Part model, mm, in its own coordinate system. Face numbers are marked on the shaded views. A direction names the side the tool comes from. Round coordinates to 2 decimals unless told otherwise and drop trailing zeros. Loops run counter-clockwise (first coordinate to the right, second up) from the corner with the lowest first, then second, coordinate; pieces in that order, holes last.
(1) Cut at A-A on x = 6. List the corners of the cut face in (y, z).
(2) Probe probe 1 along Z at (x, y) = (-13.5, -1.75); probe 2 along Y at (x, z) = (16, 2.25); probe 3 along X at (y, z) = (-3.5, 2.75). List the from-to ranges inside material, lowest first.
(3) Cut at B-B on y = 6.25. List the corners of the cut face in (x, z).
(4) Tool access for the marked faces 1, 2 and 3: list every direction of +Z, -Z, +X, -X, +Y, -Y with a clear straight run to the whole face (end or side of a thin tool).
(5) Cut at D-D on x = -4. List the corners of the cut face in (y, z), then the cut area to 3 significant figures.
(6) Flat gauge pins, fed straight in: pin 1 (5.5 mm diameter, centred on y = 1.5, z = 9, fed in from +X); pin 2 (6 mm diameter, centred on x = 15, z = 8.5, fed in from +Y); pin 3 (2.5 mm diameter, centred on x = -7, z = 8.5, fed in from -Y); pin 4 (3 mm diameter, centred on x = -7.5, z = 8.5, fed in from +Y). Where does each tip first touch, or does it go through?
(7) Cut at C-C on z = 10.75. List the corners of the cut face in (x, y), then the cut area to 3 significant figures.
from build123d import *

# Parameters (mm, degrees)
F0_W     = 54
F0_H     = 22.4
F0_W_2   = 5
F0_H_2   = 5
F1_DEPTH = 2
F2_DEPTH = 13
F3_DEPTH = 3.5
F4_R     = 2


# Not quite as in the source:
# - a feature names something its author has since deleted; it is built from what else it names


with BuildPart() as f1:
    # F0 (on Top) → F1 (new body)
    with BuildSketch(Plane.XY):
        with Locations((1.3893617413, 0.829365923)):
            Rectangle(F0_W, F0_H)
        Polygon((-23.1106382587, 3.1091097071), (-23.1106382587, 9.529365923), (25.8893617413, 9.529365923), (25.8893617413, 3.079365923), (25.8893617413, 0.829365923), (25.8893617413, -1.420634077), (25.8893617413, -7.870634077), (-23.1106382587, -7.870634077), (-23.1106382587, -1.3557597995), (-23.1106382587, 0.859365923), align=None, mode=Mode.SUBTRACT)
        with BuildLine():
            Line((25.8893617413, 9.529365923), (-23.1106382587, 9.529365923))
            Line((-23.1106382587, 9.529365923), (-23.1106382587, 3.1091097071))
            Line((-23.1106382587, 3.1091097071), (-20.8945927259, 3.1091097071))
            ThreePointArc((-20.8945927259, 3.1091097071), (-19.2816983534, 2.4623159458), (-18.6106382587, 0.859365923))
            ThreePointArc((-18.6106382587, 0.859365923), (-19.4158848712, -0.8655073041), (-21.2552495026, -1.3557597995))
            Line((-21.2552495026, -1.3557597995), (-23.1106382587, -1.3557597995))
            Line((-23.1106382587, -1.3557597995), (-23.1106382587, -7.870634077))
            Line((-23.1106382587, -7.870634077), (25.8893617413, -7.870634077))
            Line((25.8893617413, -7.870634077), (25.8893617413, -1.420634077))
            Line((25.8893617413, -1.420634077), (23.6393617413, -1.420634077))
            ThreePointArc((23.6393617413, -1.420634077), (21.3893617413, 0.829365923), (23.6393617413, 3.079365923))
            Line((23.6393617413, 3.079365923), (25.8893617413, 3.079365923))
            Line((25.8893617413, 3.079365923), (25.8893617413, 9.529365923))
        make_face()
        with Locations((-5.8658428788, 0.829365923)):
            Rectangle(F0_W_2, F0_H_2, mode=Mode.SUBTRACT)
        with BuildLine():
            Line((-20.8945927259, 3.1091097071), (-23.1106382587, 3.1091097071))
            Line((-23.1106382587, 3.1091097071), (-23.1106382587, 0.859365923))
            ThreePointArc((-23.1106382587, 0.859365923), (-22.4635882815, 2.4383058282), (-20.8945927259, 3.1091097071))
        make_face()
        with BuildLine():
            Line((25.8893617413, 0.829365923), (25.8893617413, 3.079365923))
            Line((25.8893617413, 3.079365923), (23.6393617413, 3.079365923))
            ThreePointArc((23.6393617413, 3.079365923), (25.230351999, 2.4203561806), (25.8893617413, 0.829365923))
        make_face()
        with BuildLine():
            ThreePointArc((-21.2552495026, -1.3557597995), (-22.5855114857, -0.5853874645), (-23.1106382587, 0.859365923))
            Line((-23.1106382587, 0.859365923), (-23.1106382587, -1.3557597995))
            Line((-23.1106382587, -1.3557597995), (-21.2552495026, -1.3557597995))
        make_face()
        with BuildLine():
            ThreePointArc((-20.8945927259, 3.1091097071), (-22.4635882815, 2.4383058282), (-23.1106382587, 0.859365923))
            ThreePointArc((-23.1106382587, 0.859365923), (-22.5855114857, -0.5853874645), (-21.2552495026, -1.3557597995))
            Line((-21.2552495026, -1.3557597995), (-20.8945927259, -1.3557597995))
            Line((-20.8945927259, -1.3557597995), (-20.8945927259, -0.5963975782))
            ThreePointArc((-20.8945927259, -0.5963975782), (-22.8606382587, 0.829365923), (-20.8945927259, 2.2551294242))
            Line((-20.8945927259, 2.2551294242), (-20.8945927259, 3.1091097071))
        make_face()
        with BuildLine():
            ThreePointArc((-18.6106382587, 0.859365923), (-19.2816983534, 2.4623159458), (-20.8945927259, 3.1091097071))
            Line((-20.8945927259, 3.1091097071), (-20.8945927259, 2.2551294242))
            ThreePointArc((-20.8945927259, 2.2551294242), (-20.1463342813, 1.7099713115), (-19.8606382587, 0.829365923))
            ThreePointArc((-19.8606382587, 0.829365923), (-20.1463342813, -0.0512394656), (-20.8945927259, -0.5963975782))
            Line((-20.8945927259, -0.5963975782), (-20.8945927259, -1.3557597995))
            Line((-20.8945927259, -1.3557597995), (-21.2552495026, -1.3557597995))
            ThreePointArc((-21.2552495026, -1.3557597995), (-19.4158848712, -0.8655073041), (-18.6106382587, 0.859365923))
        make_face()
        with BuildLine():
            ThreePointArc((23.6393617413, -1.420634077), (25.230351999, -0.7616243347), (25.8893617413, 0.829365923))
            ThreePointArc((25.8893617413, 0.829365923), (25.230351999, 2.4203561806), (23.6393617413, 3.079365923))
            Line((23.6393617413, 3.079365923), (23.6393617413, 2.2174858052))
            ThreePointArc((23.6393617413, 2.2174858052), (25.043666155, 2.0748896863), (25.7078010014, 0.829365923))
            ThreePointArc((25.7078010014, 0.829365923), (25.043666155, -0.4161578404), (23.6393617413, -0.5587539593))
            Line((23.6393617413, -0.5587539593), (23.6393617413, -1.420634077))
        make_face()
        with BuildLine():
            Line((25.8893617413, -1.420634077), (25.8893617413, 0.829365923))
            ThreePointArc((25.8893617413, 0.829365923), (25.230351999, -0.7616243347), (23.6393617413, -1.420634077))
            Line((23.6393617413, -1.420634077), (25.8893617413, -1.420634077))
        make_face()
        with BuildLine():
            Line((23.6393617413, 2.2174858052), (23.6393617413, 3.079365923))
            ThreePointArc((23.6393617413, 3.079365923), (21.3893617413, 0.829365923), (23.6393617413, -1.420634077))
            Line((23.6393617413, -1.420634077), (23.6393617413, -0.5587539593))
            ThreePointArc((23.6393617413, -0.5587539593), (22.7078010014, 0.829365923), (23.6393617413, 2.2174858052))
        make_face()
        with Locations((-5.8658428788, 0.829365923)):
            Rectangle(F0_W_2, F0_H_2)
    extrude(amount=F1_DEPTH)

    # F0 (on Top) → F2 (join)
    with BuildSketch(Plane.XY):
        with Locations((-5.8658428788, 0.829365923)):
            Rectangle(F0_W_2, F0_H_2)
    extrude(amount=F2_DEPTH)

    # F0 (on Top) → F3 (join)
    with BuildSketch(Plane.XY):
        with BuildLine():
            Line((25.8893617413, 9.529365923), (-23.1106382587, 9.529365923))
            Line((-23.1106382587, 9.529365923), (-23.1106382587, 3.1091097071))
            Line((-23.1106382587, 3.1091097071), (-20.8945927259, 3.1091097071))
            ThreePointArc((-20.8945927259, 3.1091097071), (-19.2816983534, 2.4623159458), (-18.6106382587, 0.859365923))
            ThreePointArc((-18.6106382587, 0.859365923), (-19.4158848712, -0.8655073041), (-21.2552495026, -1.3557597995))
            Line((-21.2552495026, -1.3557597995), (-23.1106382587, -1.3557597995))
            Line((-23.1106382587, -1.3557597995), (-23.1106382587, -7.870634077))
            Line((-23.1106382587, -7.870634077), (25.8893617413, -7.870634077))
            Line((25.8893617413, -7.870634077), (25.8893617413, -1.420634077))
            Line((25.8893617413, -1.420634077), (23.6393617413, -1.420634077))
            ThreePointArc((23.6393617413, -1.420634077), (21.3893617413, 0.829365923), (23.6393617413, 3.079365923))
            Line((23.6393617413, 3.079365923), (25.8893617413, 3.079365923))
            Line((25.8893617413, 3.079365923), (25.8893617413, 9.529365923))
        make_face()
        with Locations((-5.8658428788, 0.829365923)):
            Rectangle(F0_W_2, F0_H_2, mode=Mode.SUBTRACT)
        with Locations((-5.8658428788, 0.829365923)):
            Rectangle(F0_W_2, F0_H_2)
    extrude(amount=F3_DEPTH)

    # F4
    f4_edges = [f1.edges().sort_by_distance(p)[0] for p in [
        (-25.610638, 12.029366, 1),
        (-25.610638, -10.370634, 1),
        (28.389362, 12.029366, 1),
        (28.389362, -10.370634, 1),
    ]]
    fillet(f4_edges, radius=F4_R)


solid = f1.part
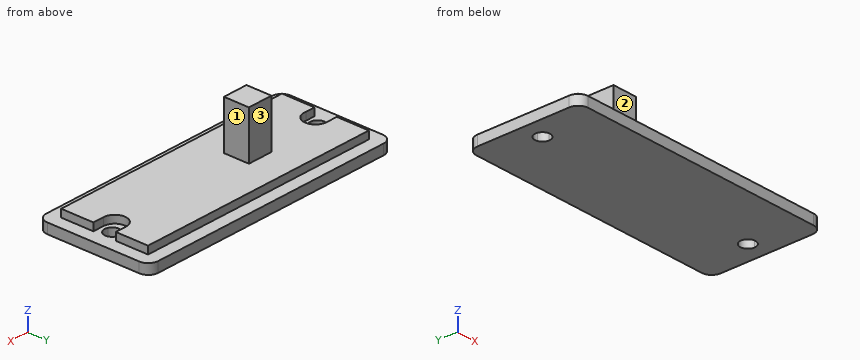
Final values:
1. outline: (-10.37, 0) - (12.03, 0) - (12.03, 2) - (9.53, 2) - (9.53, 3.5) - (-7.87, 3.5) - (-7.87, 2) - (-10.37, 2) - close
2. probe 1: z = 0 to 3.5
2. probe 2: y = -7.87 to 9.53
2. probe 3: x = -23.11 to 25.89
3. outline: (-25.61, 0) - (28.39, 0) - (28.39, 2) - (25.89, 2) - (25.89, 3.5) - (-23.11, 3.5) - (-23.11, 2) - (-25.61, 2) - close
4. face 1: +Z, +X, +Y, -Y
4. face 2: +Z, +X, -X, -Y
4. face 3: +Z, +X, -X, +Y
5. outline: (-10.37, 0) - (12.03, 0) - (12.03, 2) - (9.53, 2) - (9.53, 3.5) - (3.33, 3.5) - (3.33, 13) - (-1.67, 13) - (-1.67, 3.5) - (-7.87, 3.5) - (-7.87, 2) - (-10.37, 2) - close
5. area: 118 mm2
6. pin 1: stops at x = -3.37
6. pin 2: passes through
6. pin 3: stops at y = -1.67
6. pin 4: stops at y = 3.33
7. outline: (-8.37, -1.67) - (-3.37, -1.67) - (-3.37, 3.33) - (-8.37, 3.33) - close
7. area: 25.0 mm2
